Work out the finished part from the listing and answer in its coordinate system (mm). A direction names the side the tool comes from. Give positions to 0.01 mm unless a question says otherwise; leave off trailing zeros. Order: outer loops, then holes, each group sorted by start corner. A loop starts at its lowest first (then second) coordinate and runs counter-clockwise, first axis right, second up.
```python
from build123d import *

# Parameters (mm, degrees)
SKETCH1_W            = 281.94
SKETCH1_H            = 228.6
BOSS_EXTRUDE2_DEPTH  = 25.4
SKETCH3_W            = 281.94
SKETCH3_H            = 17.526
CUT_EXTRUDE1_DEPTH   = 8.128
SKETCH4_W            = 11.43
SKETCH4_H            = 211.074
BOSS_EXTRUDE4_DEPTH  = 3.175
SKETCH5_W            = 278.765
SKETCH5_H            = 11.43
BOSS_EXTRUDE9_DEPTH  = 3.175
SKETCH9_W            = 11.43
SKETCH9_H            = 207.899
BOSS_EXTRUDE10_DEPTH = 3.175
SKETCH8_W            = 281.94
SKETCH8_H            = 11.43
BOSS_EXTRUDE11_DEPTH = 3.175


with BuildPart() as part:
    # Sketch1 → Boss-Extrude2 (new body)
    with BuildSketch(Plane.XY):
        with Locations((72.606829268, 16.339634146)):
            Rectangle(SKETCH1_W, SKETCH1_H)
    extrude(amount=BOSS_EXTRUDE2_DEPTH)

    # Sketch3 → Cut-Extrude1 (cut)
    with BuildSketch(Plane.XY.offset(25.4)):
        with Locations((72.606829268, -89.197365854)):
            Rectangle(SKETCH3_W, SKETCH3_H)
    extrude(amount=-CUT_EXTRUDE1_DEPTH, mode=Mode.SUBTRACT)



with BuildPart() as body_2:
    # Sketch4 → Boss-Extrude4 (new body)
    with BuildSketch(Plane.ZY.offset(68.363170732)):
        with Locations((31.115, 25.102634146)):
            Rectangle(SKETCH4_W, SKETCH4_H)
    extrude(amount=-BOSS_EXTRUDE4_DEPTH)


with BuildPart() as part_1:
    add(part.part)

    add(body_2.part)  # Boss-Extrude9 merges body 2
    # Sketch5 → Boss-Extrude9 (add)
    with BuildSketch(Plane(origin=(0, 130.639634146, 0), x_dir=(1, 0, 0), z_dir=(0, 1, 0))):
        with Locations((74.194329268, -31.115)):
            Rectangle(SKETCH5_W, SKETCH5_H)
    extrude(amount=-BOSS_EXTRUDE9_DEPTH)

    # Sketch9 → Boss-Extrude10 (add)
    with BuildSketch(Plane(origin=(213.576829268, 0, 0), x_dir=(0, 0, -1), z_dir=(1, 0, 0))):
        with Locations((-31.115, 23.515134146)):
            Rectangle(SKETCH9_W, SKETCH9_H)
    extrude(amount=-BOSS_EXTRUDE10_DEPTH)


with BuildPart() as body_2_2:
    # Sketch8 → Boss-Extrude11 (new body)
    with BuildSketch(Plane.XZ.offset(97.960365854)):
        with Locations((72.606829268, 22.987)):
            Rectangle(SKETCH8_W, SKETCH8_H)
    extrude(amount=-BOSS_EXTRUDE11_DEPTH)

    # Combine1: union part
    add(part_1.part)


solid = body_2_2.part
```
1. The mould has two halves that part along Y. Classify faces 1 (the face through (71, 130.64, 18)), 2 (the face through (71, -88, 17.272)), 3 (the face through (-68.363, 18, 18)): pulls with the +Y half, pulls with the -Y half, needs draft (parallel to the pull), parting line crosses it, or undercut.
Findings below:
face 1: pulls with the +Y half
face 2: undercut
face 3: needs draft
2. Which of the six approach directions +Z, -Z, +X, -X, +Y, -Y give full straight-line access (tool end or side, diameter ignored) to faces 4 (the face through (75, -80.434, 23)), 5 (the face through (71, 127.465, 31)), 6 (the face through (71, 18, 0))?
Findings below:
face 4: +Z, +X, -X
face 5: +Z
face 6: -Z, +X, -X, +Y, -Y
3. The part is cut by section A-A (y = 90.5). Write down the section's boundary in (x, z), then the cut area to 3 significant figures.
Findings below:
outline: (-68.36, 0) - (213.58, 0) - (213.58, 36.83) - (210.4, 36.83) - (210.4, 25.4) - (-65.19, 25.4) - (-65.19, 36.83) - (-68.36, 36.83) - close
area: 7,230 mm2
4. Straight lines are drawn through the part: probe 1 along Y at (x, z) = (-0.5, 20.5); probe 2 along Y at (x, z) = (-20, 25.5); probe 3 along X at (y, z) = (31.5, 28). For each, find the intervals that lie inside material, in ascending order.
Findings below:
probe 1: y = -97.96 to -94.79, -80.43 to 130.64
probe 2: y = -97.96 to -94.79, 127.46 to 130.64
probe 3: x = -68.36 to -65.19, 210.4 to 213.58
5. Given P1, Ø12, axis at x = 14.5, z = 32.5, coming from the -Y side; P2, Ø4, axis at x = 66, y = -48.5, coming from the +Z side; P3, Ø1, axis at x = 83.5, y = -96, coming from the +Z side, each flat-ended and moving along its own axis, determine where each tip first touches the part or whether it passes through.
Findings below:
P1: stops at y = -97.96
P2: stops at z = 25.4
P3: stops at z = 28.7
6. The part is cut by section B-B (x = -44). Write down the section's boundary in (y, z), then the cut area to 3 significant figures.
Findings below:
outline: (-97.96, 0) - (130.64, 0) - (130.64, 36.83) - (127.46, 36.83) - (127.46, 25.4) - (-80.43, 25.4) - (-80.43, 17.27) - (-94.79, 17.27) - (-94.79, 28.7) - (-97.96, 28.7) - close
area: 5,740 mm2
